Part print with two shaded views. Sizes in mm from the minimum x, y, z corner. A direction names the side the tool comes from. Give positions to 0.01 mm unless a question says otherwise; leave off trailing zeros. Loops run counter-clockwise (first coordinate to the right, second up) from the corner with the lowest first, then second, coordinate; pieces in that order, holes last. Notation, with made-up numbers: (-10, 63) -> (-5, 63) arc R17 cw to (-5, 79) -> close; hole circle Ø9 at (42, 79). An arc over 180 degrees is marked (long way). One line per question, with ' | ' between items. Start each with the question number.
(1) Flat gauge pins, fed straight in: pin 1 Ø4 at (y, z) = (23, 9.5) entering from -X; pin 2 Ø6 at (y, z) = (49, 11) entering from +X; pin 3 Ø1 at (x, y) = (49.5, 41.5) entering from +Z; pin 4 Ø6 at (x, z) = (3.5, 7.5) entering from -Y. Where does each tip first touch, or does it go through?
(2) 3-axis set-ups, long thin cutter, end or side, ignore diameter. For the marked faces 4, 5, 6 and 7: which of +Z, -Z, +X, -X, +Y, -Y reach the whole face in a straight line?
(3) Mould opens along Y. For the marked faces 1, 2 and 3 say: pulls with the +Y half, pulls with the -Y half, needs draft (parallel to the pull), parting line crosses it, or undercut.
(4) Drill centre lines: L1, parallel to X at y = 20.5, z = 12.25; L2, parallel to X at y = 47, z = 17.75. Where is each one in solid material? Low to high. Write a range as from..to.
(5) Slice it at D-D, the plane x = 6. Write the cut outline in (y, z).
(6) Slice it at A-A, the plane x = 25. Write the cut outline in (y, z), then the cut area to 3 significant figures.
(7) Slice it at C-C, the plane z = 9.25. Write the cut outline in (x, y), then the cut area to 3 significant figures.
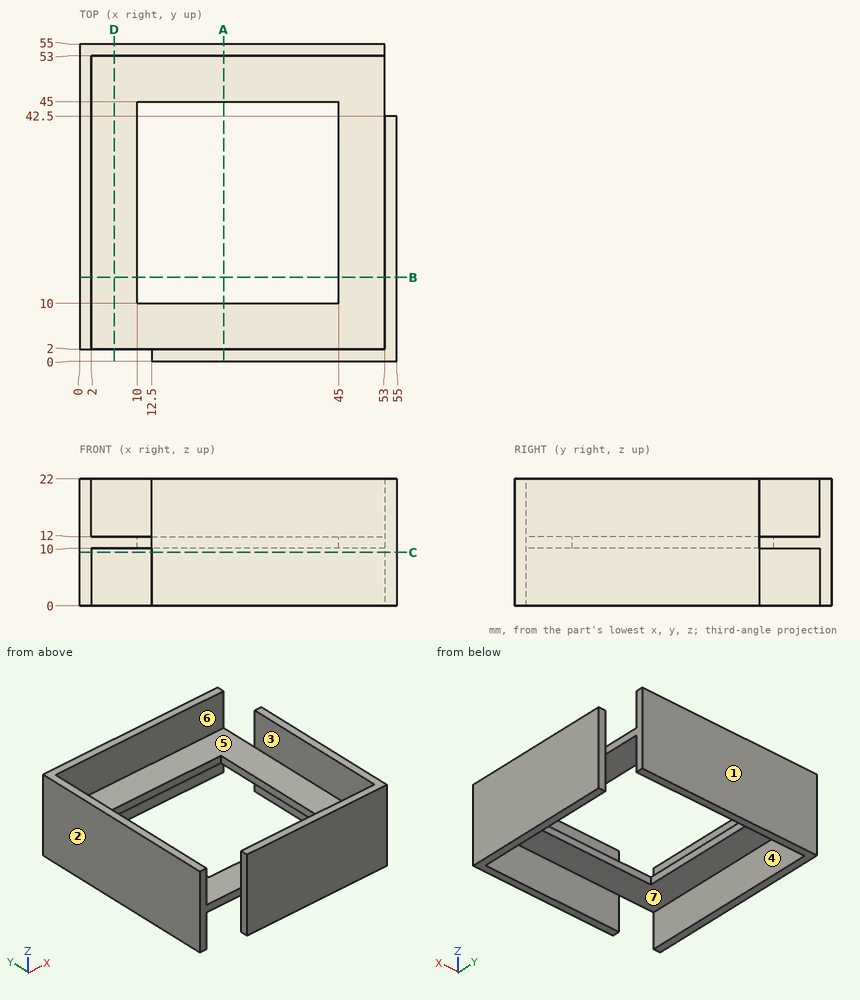
Final values:
1) pin 1: x = 0 | pin 2: x = 53 | pin 3: z = 12 | pin 4: y = 2
2) face 4: -Z, -Y | face 5: +Z | face 6: +Z, +X | face 7: -Z
3) face 1: pulls with the +Y half | face 2: needs draft | face 3: undercut
4) L1: 0..2, 53..55 | L2: 0..2
5) outline: (2, 10) -> (53, 10) -> (53, 0) -> (55, 0) -> (55, 22) -> (53, 22) -> (53, 12) -> (2, 12) -> close
6) outline: (0, 0) -> (2, 0) -> (2, 10) -> (10, 10) -> (10, 12) -> (2, 12) -> (2, 22) -> (0, 22) -> close; (45, 10) -> (53, 10) -> (53, 0) -> (55, 0) -> (55, 22) -> (53, 22) -> (53, 12) -> (45, 12) -> close | area: 120 mm2
7) outline: (0, 2) -> (2, 2) -> (2, 53) -> (53, 53) -> (53, 55) -> (0, 55) -> close; (12.5, 0) -> (55, 0) -> (55, 42.5) -> (53, 42.5) -> (53, 2) -> (12.5, 2) -> close | area: 374 mm2
